Source: CAD feature listing. Evaluate the final solid. Frame: model axes, mm. A direction names the side the tool comes from. Give positions to 0.01 mm unless a question says otherwise; leave off trailing zeros. Loops run counter-clockwise (first coordinate to the right, second up) from the corner with the lowest first, then second, coordinate; pieces in that order, holes last. Notation, with made-up numbers: M 82,3.5 L 137,3.5 A21 ccw 137,32.5 Z; hole C 6,58 d8. An arc over 180 degrees is marked long. Put each result on its own line as item: value.
from build123d import *

# Parameters (mm, degrees)
BOSS_EXTRUDE1_DEPTH = 25.4


with BuildPart() as part:
    # Sketch1 → Boss-Extrude1 (new body)
    with BuildSketch(Plane.XY):
        Polygon((-45.000100804, -22.499999999), (44.999899202, -22.499999999), (44.999899202, 22.5), (26.749899972, 22.5), (26.749899972, 17.999999372), (29.299918194, 17.999999372), (29.299918002, 9.200011166), (27.299917722, 7.200011061), (17.699911829, 7.200011271), (15.699911706, 9.200011568), (15.699911899, 17.999999102), (18.249899884, 17.999999102), (18.249899884, 22.5), (-18.250100028, 22.5), (-18.250100028, 17.999999372), (-15.700081806, 17.999999372), (-15.700081998, 9.200011166), (-17.700082278, 7.200011061), (-27.300088171, 7.200011271), (-29.300088294, 9.200011568), (-29.300088101, 17.999999102), (-26.750100116, 17.999999102), (-26.750100116, 22.5), (-45.000100804, 22.5), (-45.000100804, 4.250000064), (-40.500099403, 4.250000064), (-40.500099403, 6.800018286), (-31.700111197, 6.800018094), (-29.700111092, 4.800017814), (-29.700111302, -4.79998808), (-31.700111599, -6.799988202), (-40.500099133, -6.79998801), (-40.500099133, -4.250000024), (-45.000100804, -4.250000024), align=None)
        with BuildLine():
            Line((19.237162182, 1.848524255), (17.903705922, 3.181980515))
            Line((17.903705922, 3.181980515), (19.317919485, 4.596194078))
            Line((19.317919485, 4.596194078), (20.651375745, 3.262737818))
            ThreePointArc((20.651375745, 3.262737818), (22.4999, 3.749999999), (24.348424255, 3.262737818))
            Line((24.348424255, 3.262737818), (25.681880515, 4.596194078))
            Line((25.681880515, 4.596194078), (27.096094078, 3.181980515))
            Line((27.096094078, 3.181980515), (25.762637818, 1.848524255))
            ThreePointArc((25.762637818, 1.848524255), (26.249899999, 0), (25.762637818, -1.848524255))
            Line((25.762637818, -1.848524255), (27.096094078, -3.181980515))
            Line((27.096094078, -3.181980515), (25.681880515, -4.596194078))
            Line((25.681880515, -4.596194078), (24.348424255, -3.262737818))
            ThreePointArc((24.348424255, -3.262737818), (22.4999, -3.749999999), (20.651375745, -3.262737818))
            Line((20.651375745, -3.262737818), (19.317919483, -4.596194079))
            Line((19.317919483, -4.596194079), (17.90370592, -3.181980517))
            Line((17.90370592, -3.181980517), (19.237162182, -1.848524255))
            ThreePointArc((19.237162182, -1.848524255), (18.749900001, 0), (19.237162182, 1.848524255))
        make_face(mode=Mode.SUBTRACT)
        with BuildLine():
            Line((-25.682080517, -4.596194079), (-27.09629408, -3.181980517))
            Line((-27.09629408, -3.181980517), (-25.762837818, -1.848524255))
            ThreePointArc((-25.762837818, -1.848524255), (-26.250099999, 0), (-25.762837818, 1.848524255))
            Line((-25.762837818, 1.848524255), (-27.096294078, 3.181980515))
            Line((-27.096294078, 3.181980515), (-25.682080515, 4.596194078))
            Line((-25.682080515, 4.596194078), (-24.348624255, 3.262737818))
            ThreePointArc((-24.348624255, 3.262737818), (-22.5001, 3.749999999), (-20.651575745, 3.262737818))
            Line((-20.651575745, 3.262737818), (-19.318119485, 4.596194078))
            Line((-19.318119485, 4.596194078), (-17.903905922, 3.181980515))
            Line((-17.903905922, 3.181980515), (-19.237362182, 1.848524255))
            ThreePointArc((-19.237362182, 1.848524255), (-18.750100001, 0), (-19.237362182, -1.848524255))
            Line((-19.237362182, -1.848524255), (-17.903905922, -3.181980515))
            Line((-17.903905922, -3.181980515), (-19.318119485, -4.596194078))
            Line((-19.318119485, -4.596194078), (-20.651575745, -3.262737818))
            ThreePointArc((-20.651575745, -3.262737818), (-22.5001, -3.749999999), (-24.348624255, -3.262737818))
            Line((-24.348624255, -3.262737818), (-25.682080517, -4.596194079))
        make_face(mode=Mode.SUBTRACT)
        Polygon((42.999881918, 20.500011944), (42.999881663, 8.8), (31.299899711, 8.8), (31.299899711, 20.5000122), align=None, mode=Mode.SUBTRACT)
        Polygon((42.999881952, -20.5), (31.2999, -20.5), (31.2999, -8.7999878), (42.999882208, -8.799988056), align=None, mode=Mode.SUBTRACT)
        Polygon((-31.300117792, -8.799988056), (-31.300118048, -20.5), (-43.0001, -20.5), (-43.0001, -8.7999878), align=None, mode=Mode.SUBTRACT)
        Polygon((-31.300118048, 8.8), (-43.0001, 8.8), (-43.0001, 20.5000122), (-31.300117792, 20.500011944), align=None, mode=Mode.SUBTRACT)
        with BuildLine():
            Line((-26.750099976, -22.200012315), (-26.750099976, -17.999999113))
            Line((-26.750099976, -17.999999113), (-29.300118194, -17.999999113))
            Line((-29.300118194, -17.999999113), (-29.300118002, -9.200011166))
            Line((-29.300118002, -9.200011166), (-27.300117722, -7.200011061))
            Line((-27.300117722, -7.200011061), (-17.700111829, -7.200011271))
            Line((-17.700111829, -7.200011271), (-15.700111706, -9.200011568))
            Line((-15.700111706, -9.200011568), (-15.700111899, -17.999998844))
            Line((-15.700111899, -17.999998844), (-18.250099887, -17.999998844))
            Line((-18.250099887, -17.999998844), (-18.250099887, -22.20001241))
            Line((-18.250099887, -22.20001241), (-18.550118283, -22.20001241))
            Line((-18.550118283, -22.20001241), (-19.017895639, -21.73223406))
            ThreePointArc((-19.017895639, -21.73223406), (-19.828954662, -21.190300811), (-20.785664471, -20.999999134))
            Line((-20.785664471, -20.999999134), (-24.214566009, -20.999999134))
            ThreePointArc((-24.214566009, -20.999999134), (-25.171313387, -21.190316374), (-25.982392349, -21.732291572))
            Line((-25.982392349, -21.732291572), (-26.450081665, -22.200012315))
            Line((-26.450081665, -22.200012315), (-26.750099976, -22.200012315))
        make_face(mode=Mode.SUBTRACT)
        with BuildLine():
            Line((18.249900024, -22.200012315), (18.249900024, -17.999999113))
            Line((18.249900024, -17.999999113), (15.699881806, -17.999999113))
            Line((15.699881806, -17.999999113), (15.699881998, -9.200011166))
            Line((15.699881998, -9.200011166), (17.699882278, -7.200011061))
            Line((17.699882278, -7.200011061), (27.299888171, -7.200011271))
            Line((27.299888171, -7.200011271), (29.299888294, -9.200011568))
            Line((29.299888294, -9.200011568), (29.299888101, -17.999998844))
            Line((29.299888101, -17.999998844), (26.749900113, -17.999998844))
            Line((26.749900113, -17.999998844), (26.749900113, -22.20001241))
            Line((26.749900113, -22.20001241), (26.449881717, -22.20001241))
            Line((26.449881717, -22.20001241), (25.982104361, -21.73223406))
            ThreePointArc((25.982104361, -21.73223406), (25.171045338, -21.190300811), (24.214335529, -20.999999134))
            Line((24.214335529, -20.999999134), (20.785433991, -20.999999134))
            ThreePointArc((20.785433991, -20.999999134), (19.828686613, -21.190316374), (19.017607651, -21.732291572))
            Line((19.017607651, -21.732291572), (18.549918335, -22.200012315))
            Line((18.549918335, -22.200012315), (18.249900024, -22.200012315))
        make_face(mode=Mode.SUBTRACT)
        with BuildLine():
            Line((31.699911166, -6.800018002), (29.699911061, -4.800017722))
            Line((29.699911061, -4.800017722), (29.699911271, 4.799988171))
            Line((29.699911271, 4.799988171), (31.699911568, 6.799988294))
            Line((31.699911568, 6.799988294), (40.499898813, 6.799988101))
            Line((40.499898813, 6.799988101), (40.499898813, 4.250000116))
            Line((40.499898813, 4.250000116), (44.69991241, 4.250000116))
            Line((44.69991241, 4.250000116), (44.69991241, 3.949981717))
            Line((44.69991241, 3.949981717), (44.23213406, 3.482204361))
            ThreePointArc((44.23213406, 3.482204361), (43.690200811, 2.671145338), (43.499899134, 1.714435529))
            Line((43.499899134, 1.714435529), (43.499899134, -1.714466009))
            ThreePointArc((43.499899134, -1.714466009), (43.690216374, -2.671213387), (44.232191572, -3.482292349))
            Line((44.232191572, -3.482292349), (44.699912315, -3.949981665))
            Line((44.699912315, -3.949981665), (44.699912315, -4.249999976))
            Line((44.699912315, -4.249999976), (40.499899113, -4.249999976))
            Line((40.499899113, -4.249999976), (40.499899113, -6.800018194))
            Line((40.499899113, -6.800018194), (31.699911166, -6.800018002))
        make_face(mode=Mode.SUBTRACT)
        Polygon((13.699911396, 20.5), (13.699911131, 8.37158507), (15.4999, 6.571596043), (15.4999, -6.571596043), (13.699910134, -8.371586067), (13.699910399, -20.5), (-13.7001122, -20.5), (-13.700111724, -8.371584476), (-15.5001, -6.571596043), (-15.5001, 6.571596848), (-13.700112474, 8.371584531), (-13.700112739, 20.5), align=None, mode=Mode.SUBTRACT)
    extrude(amount=BOSS_EXTRUDE1_DEPTH)


solid = part.part
1. Section query D-D (z = 8.25). State how many separate pieces and enclosed holes the cut face has, plus the area to 3 significant figures.
Found:
separate pieces: 1
enclosed holes: 10
area: 1,150 mm^2
2. Section query C-C (x = 7). Output: boundary loops of the cut face in (y, z), plus the area to 3 significant figures.
Found:
outline: M -22.5,0 L -20.5,0 L -20.5,25.4 L -22.5,25.4 Z; M 20.5,0 L 22.5,0 L 22.5,25.4 L 20.5,25.4 Z
area: 102 mm^2
3. Draft query along X for faces 1 (the flat face through (-45, -13, 13)), 2 (the flat face through (-36, 22.5, 13)), 3 (the flat face through (29.3, 14, 13)). Return one class per face: pulls with the +X half, pulls with the -X half, needs draft (parallel to the pull), parting line crosses it, or undercut.
Found:
face 1: pulls with the -X half
face 2: needs draft
face 3: undercut
4. Contact query for flat-ended pins moving along their axis: P1, Ø3, axis at x = 20.5, z = 8, coming from the +Y side; P2, Ø8, axis at x = 27, y = 2, coming from the -Z side; P3, Ø2.5, axis at y = -1, z = 16.5, coming from the -X side. Output: stop coordinate, or through.
Found:
P1: y = 7.2
P2: z = 0
P3: x = -29.7
5. Section query A-A (y = 11.5). Output: boundary loops of the cut face in (x, z), plus the area to 3 significant figures.
Found:
outline: M -45,0 L -43,0 L -43,25.4 L -45,25.4 Z; M -31.3,0 L -29.3,0 L -29.3,25.4 L -31.3,25.4 Z; M -15.7,0 L -13.7,0 L -13.7,25.4 L -15.7,25.4 Z; M 13.7,0 L 15.7,0 L 15.7,25.4 L 13.7,25.4 Z; M 29.3,0 L 31.3,0 L 31.3,25.4 L 29.3,25.4 Z; M 43,0 L 45,0 L 45,25.4 L 43,25.4 Z
area: 305 mm^2
6. Access query for faces 4 (the flat face through (45, 0, 13)), 5 (the flat face through (36, 6.8, 13)), 6 (the flat face through (18.25, 20, 13)). Directions: +Z, -Z, +X, -X, +Y, -Y. A direction counts if a zero-diameter tool reaches every point of the face in a straight line with its end or side. Return the directions, or none.
Found:
face 4: +Z, -Z, +X, +Y, -Y
face 5: +Z, -Z
face 6: +Z, -Z, +Y
7. Section query B-B (x = 39). Output: boundary loops of the cut face in (y, z), plus the area to 3 significant figures.
Found:
outline: M -22.5,0 L -20.5,0 L -20.5,25.4 L -22.5,25.4 Z; M -8.8,0 L -6.8,0 L -6.8,25.4 L -8.8,25.4 Z; M 6.8,0 L 8.8,0 L 8.8,25.4 L 6.8,25.4 Z; M 20.5,0 L 22.5,0 L 22.5,25.4 L 20.5,25.4 Z
area: 203 mm^2
8. Material intervals for line 1 (X direction, y = -12, z = 13.5); line 2 (Y direction, x = 41.5, z = 7.5); line 3 (X direction, y = 21, z = 9.75), sorted ascending. Write a range as from..to.
Found:
line 1: -45..-43, -31.3..-29.3, -15.7..-13.7, 13.7..15.7, 29.3..31.3, 43..45
line 2: -22.5..-20.5, -8.8..-4.25, 4.25..8.8, 20.5..22.5
line 3: -45..-26.75, -18.25..18.25, 26.75..45
